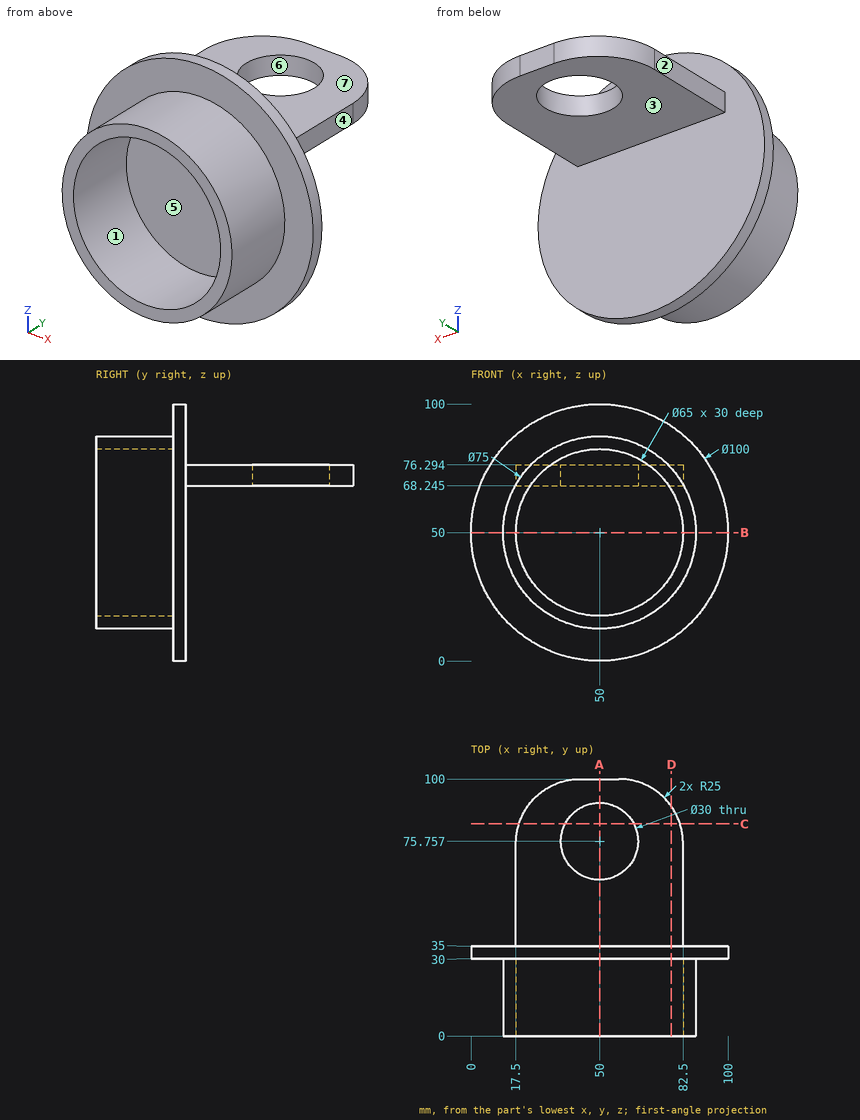
Geometry check sheet. Reference: drawing and pictorial views, mm from the part's lowest x, y, z. A direction names the side the tool comes from. Round coordinates to 2 decimals unless told otherwise and drop trailing zeros. Loops run counter-clockwise (first coordinate to the right, second up) from the corner with the lowest first, then second, coordinate; pieces in that order, holes last. Notation, with made-up numbers: (-22, -27.5) -> (30, -27.5) arc R19 cw to (30, 9.5) -> close; hole circle Ø9 at (-29.5, 42). An arc over 180 degrees is marked (long way). Answer as a JSON object with one key per item and string values. Group by question number.
Item 1: Cross-section at B-B, the plane z = 50. Record the cut outline in (x, y), plus the area to 3 significant figures.
Item 2: Release check for a two-part mould opening along Y. For the marked faces 5, 6 and 7 record: pulls with the +Y half, pulls with the -Y half, needs draft (parallel to the pull), parting line crosses it, or undercut.
Item 3: Thickness scan on line 1 along X through (y, z) = (7, 50); line 2 along Y through (x, z) = (50, 73); line 3 along Z through (x, y) = (36, 49) (1 decimal). Record the ranges inside material, lowest first.
Item 4: Cross-section at A-A, the plane x = 50. Record the cut outline in (y, z) (1 decimal).
Item 5: Cross-section at C-C, the plane y = 82.5. Record the cut outline in (x, z) (1 decimal).
Item 6: Set-up check for the marked faces 1, 2, 3 and 4: record each of +Z, -Z, +X, -X, +Y, -Y from which the full face is reachable in a straight line by a thin tool's end or side.
Item 7: Cross-section at D-D, the plane x = 78. Record the cut outline in (y, z) (1 decimal), plus the area to 3 significant figures.
Item 8: Depth check by flat-ended pin: pin 1 Ø6 at (x, y) = (62, 37.5) entering from -Z; pin 2 Ø1.5 at (x, y) = (64.5, 36.5) entering from -Z (1 decimal); pin 3 Ø10 at (y, z) = (25.5, 51.5) entering from -X. Enter the tip coordinate at first touch or a pass-through.
Determined:
{
 "1": {"outline": "(0, 30) -> (12.5, 30) -> (12.5, 0) -> (17.5, 0) -> (17.5, 30) -> (82.5, 30) -> (82.5, 0) -> (87.5, 0) -> (87.5, 30) -> (100, 30) -> (100, 35) -> (0, 35) -> close", "area": "800 mm²"},
 "2": {"face 5": "pulls with the -Y half", "face 6": "undercut", "face 7": "needs draft"},
 "3": {"line 1": "x = 12.5 to 17.5, 82.5 to 87.5", "line 2": "y = 30 to 60.76, 90.76 to 100", "line 3": "z = 68.2 to 76.3"},
 "4": {"outline": "(0, 12.5) -> (30, 12.5) -> (30, 0) -> (35, 0) -> (35, 68.2) -> (60.8, 68.2) -> (60.8, 76.3) -> (35, 76.3) -> (35, 100) -> (30, 100) -> (30, 87.5) -> (0, 87.5) -> (0, 82.5) -> (30, 82.5) -> (30, 17.5) -> (0, 17.5) -> close; (90.8, 68.2) -> (100, 68.2) -> (100, 76.3) -> (90.8, 76.3) -> close"},
 "5": {"outline": "(18.7, 68.2) -> (36.6, 68.2) -> (36.6, 76.3) -> (18.7, 76.3) -> close; (63.4, 68.2) -> (81.3, 68.2) -> (81.3, 76.3) -> (63.4, 76.3) -> close"},
 "6": {"face 1": "-Y", "face 2": "+Z, -Z, -X, +Y", "face 3": "-Z, +X, -X, +Y", "face 4": "+Z, -Z, +X, +Y"},
 "7": {"outline": "(0, 25.1) -> (30, 25.1) -> (30, 8.6) -> (35, 8.6) -> (35, 68.2) -> (89.3, 68.2) -> (89.3, 76.3) -> (35, 76.3) -> (35, 91.4) -> (30, 91.4) -> (30, 74.9) -> (0, 74.9) -> (0, 66.5) -> (30, 66.5) -> (30, 33.5) -> (0, 33.5) -> close", "area": "1,360 mm²"},
 "8": {"pin 1": "stops at z = 1.08", "pin 2": "stops at z = 68.2", "pin 3": "stops at x = 0"}
}
